from build123d import *

# Parameters (mm, degrees)
SKETCH_1_W           = 89
SKETCH_1_H           = 37.5
EXTRUDE_1_DEPTH      = 4.5
SKETCH_2_W           = 85
SKETCH_2_H           = 33.5
CUT_EXTRUDE_1_DEPTH  = 3.5
CUT_EXTRUDE_3_DEPTH  = 4
FILLET_1_R           = 2
EXTRUDE_2_DEPTH      = 1
SKETCH_10_R          = 2.5
EXTRUDE_3_DEPTH      = 4.5
SKETCH_11_R          = 0.79
CUT_EXTRUDE_9_DEPTH  = 3
SKETCH_12_W          = 85
SKETCH_12_H          = 33.5
EXTRUDE_4_DEPTH      = 0.2
SKETCH_8_R           = 7.5
CUT_EXTRUDE_8_DEPTH  = 3
SKETCH_7_R           = 10
CUT_EXTRUDE_7_DEPTH  = 3
CUT_EXTRUDE_12_DEPTH = 3.8


with BuildPart() as part:
    # 草图1 → 凸台-拉伸1 (new body)
    with BuildSketch(Plane.XY):
        Rectangle(SKETCH_1_W, SKETCH_1_H)
    extrude(amount=EXTRUDE_1_DEPTH)

    # 草图2 → 切除-拉伸1 (cut)
    with BuildSketch(Plane(origin=(0, 0, 0), x_dir=(-1, 0, 0), z_dir=(0, 0, -1))):
        Rectangle(SKETCH_2_W, SKETCH_2_H)
    extrude(amount=-CUT_EXTRUDE_1_DEPTH, mode=Mode.SUBTRACT)

    # 草图3 → 切除-拉伸3 (cut)
    with BuildSketch(Plane(origin=(44.5, 0, 0), x_dir=(0, 0, -1), z_dir=(1, 0, 0))):
        with BuildLine():
            Line((0, 1.6), (0, -1.6))
            ThreePointArc((0, -1.6), (-1.6, 0), (0, 1.6))
        make_face()
    extrude(amount=-CUT_EXTRUDE_3_DEPTH, mode=Mode.SUBTRACT)

    # 圆角1
    fillet_1_edges = [part.edges().sort_by_distance(p)[0] for p in [
        (-44.5, 0, 4.5),
        (0, -18.75, 4.5),
        (42.5, -16.75, 1.75),
        (42.5, 16.75, 1.75),
        (-42.5, 16.75, 1.75),
        (-42.5, -16.75, 1.75),
        (44.5, 0, 4.5),
        (0, 18.75, 4.5),
        (44.5, -18.75, 2.25),
        (-44.5, -18.75, 2.25),
        (-44.5, 18.75, 2.25),
        (44.5, 18.75, 2.25),
    ]]
    fillet(fillet_1_edges, radius=FILLET_1_R)

    # 草图9 → 凸台-拉伸2 (add)
    with BuildSketch(Plane(origin=(0, 0, 0), x_dir=(-1, 0, 0), z_dir=(0, 0, -1))):
        with BuildLine():
            Line((-41.5, 17.75), (41.5, 17.75))
            ThreePointArc((41.5, 17.75), (42.914213562, 17.164213562), (43.5, 15.75))
            Line((43.5, 15.75), (43.5, -15.75))
            ThreePointArc((43.5, -15.75), (42.914213562, -17.164213562), (41.5, -17.75))
            Line((41.5, -17.75), (-41.5, -17.75))
            ThreePointArc((-41.5, -17.75), (-42.914213562, -17.164213562), (-43.5, -15.75))
            Line((-43.5, -15.75), (-43.5, -1.6))
            Line((-43.5, -1.6), (-42.5, -1.6))
            Line((-42.5, -1.6), (-42.5, -14.75))
            ThreePointArc((-42.5, -14.75), (-41.914213562, -16.164213562), (-40.5, -16.75))
            Line((-40.5, -16.75), (40.5, -16.75))
            ThreePointArc((40.5, -16.75), (41.914213562, -16.164213562), (42.5, -14.75))
            Line((42.5, -14.75), (42.5, 14.75))
            ThreePointArc((42.5, 14.75), (41.914213562, 16.164213562), (40.5, 16.75))
            Line((40.5, 16.75), (-40.5, 16.75))
            ThreePointArc((-40.5, 16.75), (-41.914213562, 16.164213562), (-42.5, 14.75))
            Line((-42.5, 14.75), (-42.5, 1.6))
            Line((-42.5, 1.6), (-43.5, 1.6))
            Line((-43.5, 1.6), (-43.5, 15.75))
            ThreePointArc((-43.5, 15.75), (-42.914213562, 17.164213562), (-41.5, 17.75))
        make_face()
    extrude(amount=EXTRUDE_2_DEPTH)

    # 草图10 → 凸台-拉伸3 (add)
    with BuildSketch(Plane(origin=(0, 0, 3.5), x_dir=(-1, 0, 0), z_dir=(0, 0, -1))):
        with Locations((39.3, -13.35)):
            Circle(SKETCH_10_R)
        with Locations((39.3, 13.35)):
            Circle(SKETCH_10_R)
        with Locations((-34.5, 13.35)):
            Circle(SKETCH_10_R)
        with Locations((-34.5, -13.35)):
            Circle(SKETCH_10_R)
    extrude(amount=EXTRUDE_3_DEPTH)

    # 草图11 → 切除-拉伸9 (cut)
    with BuildSketch(Plane(origin=(0, 0, -1), x_dir=(-1, 0, 0), z_dir=(0, 0, -1))):
        with Locations((-34.5, 13.35)):
            Circle(SKETCH_11_R)
        with Locations((-34.5, -13.35)):
            Circle(SKETCH_11_R)
        with Locations((39.3, 13.35)):
            Circle(SKETCH_11_R)
        with Locations((39.3, -13.35)):
            Circle(SKETCH_11_R)
    extrude(amount=-CUT_EXTRUDE_9_DEPTH, mode=Mode.SUBTRACT)

    # 草图12 → 凸台-拉伸4 (add)
    with BuildSketch(Plane.XY.offset(4.5)):
        Rectangle(SKETCH_12_W, SKETCH_12_H)
    extrude(amount=EXTRUDE_4_DEPTH)

    # 草图8 → 切除-拉伸8 (cut)
    with BuildSketch(Plane(origin=(0, 0, 3.5), x_dir=(-1, 0, 0), z_dir=(0, 0, -1))):
        with Locations((-1, -0.55)):
            Circle(SKETCH_8_R)
    extrude(amount=-CUT_EXTRUDE_8_DEPTH, mode=Mode.SUBTRACT)

    # 草图7 → 切除-拉伸7 (cut)
    with BuildSketch(Plane(origin=(0, 0, 3.5), x_dir=(-1, 0, 0), z_dir=(0, 0, -1))):
        with Locations((29, 0)):
            Circle(SKETCH_7_R)
    extrude(amount=-CUT_EXTRUDE_7_DEPTH, mode=Mode.SUBTRACT)

    # 草图15 → 切除-拉伸12 (cut)
    with BuildSketch(Plane(origin=(0, 0, -1), x_dir=(-1, 0, 0), z_dir=(0, 0, -1))):
        Polygon((-27.5, -18.75), (-14.5, -18.75), (-13.5, -16.75), (-28.5, -16.75), align=None)
    extrude(amount=-CUT_EXTRUDE_12_DEPTH, mode=Mode.SUBTRACT)


solid = part.part
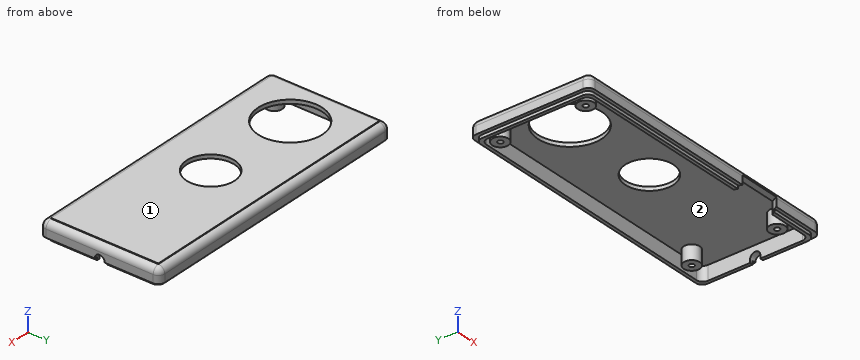
Source: CAD feature listing. Evaluate the final solid. Frame: model axes, mm. Face numbers are marked on the shaded views. Give positions to 0.01 mm unless a question says otherwise; leave off trailing zeros. Order: outer loops, then holes, each group sorted by start corner. A loop starts at its lowest first (then second) coordinate and runs counter-clockwise, first axis right, second up. Notation, with made-up numbers: (-25, -0.75) -> (-6, -0.75) arc R26 cw to (-6, 36.25) -> close; hole circle Ø10 at (77.25, 85). An arc over 180 degrees is marked (long way). Write item = value, one per line.
Q1. Cut plane C-C, the plane y = -6. Output: boundary loops of the cut face in (x, z), and give its area (3 significant figures).
Data:
outline = (-44.5, 0) -> (-43.5, 0) -> (-43.5, -1) -> (-42.5, -1) -> (-42.5, 3.5) -> (-37, 3.5) -> (-37, 4.7) -> (-42.5, 4.7) -> (-42.5, 4.5) arc R2 ccw to (-44.5, 2.5) -> close; (-21, 3.5) -> (-4.15, 3.5) -> (-4.15, 4.7) -> (-21, 4.7) -> close; (6.15, 3.5) -> (42.5, 3.5) -> (42.5, -1) -> (43.5, -1) -> (43.5, 0) -> (44.5, 0) -> (44.5, 2.5) arc R2 ccw to (42.5, 4.5) -> (42.5, 4.7) -> (6.15, 4.7) -> close
area = 88.7 mm^2
Q2. Material intervals for line 1 (Y direction, x = 34.5, z = 1.2); line 2 (X direction, y = -13, z = -0.3); line 3 (Y direction, x = 35, z = 2.8), sorted ascending. Write a range as from..to.
Data:
line_1 = -18.75..-16.75, -15.85..-14.14, -12.56..-10.85, 10.85..12.56, 14.14..15.85, 16.75..18.75
line_2 = -43.5..-42.5, -41.78..-40.01, -38.59..-36.82, 32.02..33.79, 35.21..36.98, 42.5..43.5
line_3 = -18.73..-16.75, -15.8..-10.9, 10.9..15.8, 16.75..18.73
Q3. Pin query (flat end, axial travel): pin 1 (2 mm diameter, centred on x = -16, y = 8, fed in from -Z); pin 2 (0.8 mm diameter, centred on x = -13, z = -0.5, fed in from -Y); pin 3 (9 mm diameter, centred on x = 1, y = -0.55, fed in from -Z); pin 4 (0.8 mm diameter, centred on x = -39, y = -13.5, fed in from -Z). Return the tip coordinate at first contact, or that it passes through.
Data:
pin_1 = 3.5
pin_2 = -17.75
pin_3 = through
pin_4 = 2
Q4. Pull-direction query (X, two-part tool) for the marked faces 1 and 2; classes: released by +X, released by -X, zero draft, split by the parting line, or undercut.
Data:
face_1 = zero draft
face_2 = undercut
Q5. Cut plane A-A, the plane x = 1. Output: boundary loops of the cut face in (y, z), and give its area (3 significant figures).
Data:
outline = (-18.75, 0) -> (-17.75, 0) -> (-17.75, -1) -> (-16.75, -1) -> (-16.75, 3.5) -> (-8.05, 3.5) -> (-8.05, 4.7) -> (-16.75, 4.7) -> (-16.75, 4.5) arc R2 ccw to (-18.75, 2.5) -> close; (6.95, 3.5) -> (16.75, 3.5) -> (16.75, -1) -> (17.75, -1) -> (17.75, 0) -> (18.75, 0) -> (18.75, 2.5) arc R2 ccw to (16.75, 4.5) -> (16.75, 4.7) -> (6.95, 4.7) -> close
area = 40.5 mm^2
Q6. Cut plane B-B, the plane z = 0.8. State how many separate pieces and enclosed holes the cut face has, and give its area (3 significant figures).
Data:
separate_pieces = 6
enclosed_holes = 4
area = 527 mm^2
